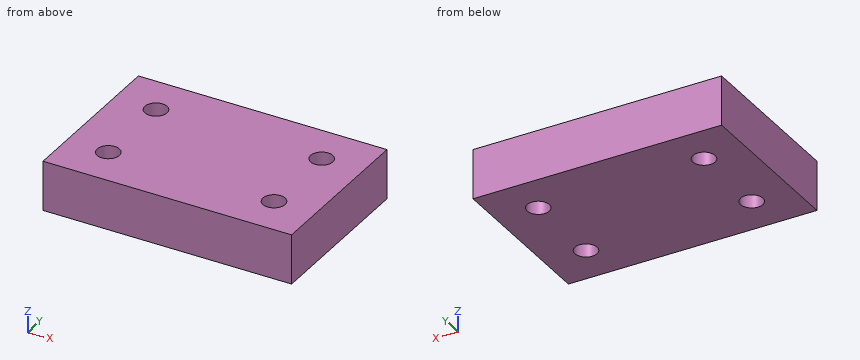
```python
from build123d import *

# Parameters (mm, degrees)
ESQUISSE1_W        = 30
ESQUISSE1_H        = 20
ESQUISSE1_R        = 1.341808551
BOSS_EXTRU_1_DEPTH = 6


with BuildPart() as part:
    # Esquisse1 → Boss.-Extru.1 (new body)
    with BuildSketch(Plane.XY):
        with Locations((15, 10)):
            Rectangle(ESQUISSE1_W, ESQUISSE1_H)
        with Locations((5, 15)):
            Circle(ESQUISSE1_R, mode=Mode.SUBTRACT)
        with Locations(Location((25, 15, 0), (0, 0, 180))):
            Circle(ESQUISSE1_R, mode=Mode.SUBTRACT)
        with Locations((25, 5)):
            Circle(ESQUISSE1_R, mode=Mode.SUBTRACT)
        with Locations(Location((5, 5, 0), (0, 0, 180))):
            Circle(ESQUISSE1_R, mode=Mode.SUBTRACT)
    extrude(amount=BOSS_EXTRU_1_DEPTH)


solid = part.part
```
The listing builds one solid part. Answer for the finished solid, in the listing's coordinates (mm). Round coordinates to 2 decimals unless told otherwise and drop trailing zeros. Order: outer loops, then holes, each group sorted by start corner. A loop starts at its lowest first (then second) coordinate and runs counter-clockwise, first axis right, second up. Notation, with made-up numbers: (-15, 3.25) - (39, 3.25) arc R24 ccw to (39, 33.25) - close; hole circle Ø5 at (61.5, -14.75). An arc over 180 degrees is marked (long way). Put each result on its own line as item: value. Start each with the question number.
(1) Find section A-A (x = 25). Give the vertices of the cut face in (y, z).
(2) Find section B-B (y = 5). Give the vertices of the cut face in (x, z).
(3) Straight lines are drawn through the part: probe 1 along Y at (x, z) = (5, 1.6); probe 2 along Y at (x, z) = (4.25, 0.4). For each, find the intervals that lie inside material, in ascending order. Write a range as from..to.
(4) Find section C-C (z = 2.4). Give the vertices of the cut face in (x, y), plus the area to 3 significant figures.
Reply:
1. outline: (0, 0) - (3.66, 0) - (3.66, 6) - (0, 6) - close; (6.34, 0) - (13.66, 0) - (13.66, 6) - (6.34, 6) - close; (16.34, 0) - (20, 0) - (20, 6) - (16.34, 6) - close
2. outline: (0, 0) - (3.66, 0) - (3.66, 6) - (0, 6) - close; (6.34, 0) - (23.66, 0) - (23.66, 6) - (6.34, 6) - close; (26.34, 0) - (30, 0) - (30, 6) - (26.34, 6) - close
3. probe 1: 0..3.66, 6.34..13.66, 16.34..20
3. probe 2: 0..3.89, 6.11..13.89, 16.11..20
4. outline: (0, 0) - (30, 0) - (30, 20) - (0, 20) - close; hole circle Ø2.68 at (5, 5); hole circle Ø2.68 at (5, 15); hole circle Ø2.68 at (25, 5); hole circle Ø2.68 at (25, 15)
4. area: 577 mm^2
